Input: part model. Units: mm. Frame: model coordinates. Face numbers are marked on the shaded views. A direction names the side the tool comes from. Round coordinates to 2 decimals unless told otherwise and drop trailing zeros. Loops run counter-clockwise (first coordinate to the right, second up) from the corner with the lowest first, then second, coordinate; pieces in that order, holes last. Notation, with made-up numbers: M 39.25,21 L 49.25,21 A7 ccw 49.25,30 Z; hole C 9.25,-1 d7. An arc over 180 degrees is marked long. Put each result on its own line as item: value. Start each with the question number.
1) Section A-A on x = -5. Output: boundary loops of the cut face in (y, z).
2) Draft query along X for the marked faces 3, 4, 5 and 6. Return one class per face: +X half, -X half, draft (parallel to the pull), parting line (faces both ways), or undercut.
3) Section B-B on z = 32.5. Output: boundary loops of the cut face in (x, y), plus the area to 3 significant figures.
4) Section C-C on y = -8. Output: boundary loops of the cut face in (x, z), plus the area to 3 significant figures.
5) Reachability of the marked faces 1 and 2 from +Z, -Z, +X, -X, +Y, -Y: full face, straight path, thin tool, end or side. Return the list, or none.
6) Line query: probe 1 along Y at (x, z) = (-5, 4); probe 2 along Y at (x, z) = (95.25, 48.2) (3 decimals); probe 3 along X at (y, z) = (-8.5, 38.5). Output: solid intervals per line, ascending.
7) Pin query (flat end, axial travel): pin 1 (5 mm diameter, centred on y = -27, z = 25.7, fed in from -X); pin 2 (6.5 mm diameter, centred on x = -5, y = -15.2, fed in from +Z); pin 3 (4.5 mm diameter, centred on y = 25, z = 48.2, fed in from +X); pin 4 (3 mm diameter, centred on y = 8.5, z = 6.5, fed in from +X). Return the tip coordinate at first contact, or that it passes through.
8) Section D-D on z = 48.2. Output: boundary loops of the cut face in (x, y) (3 decimals).
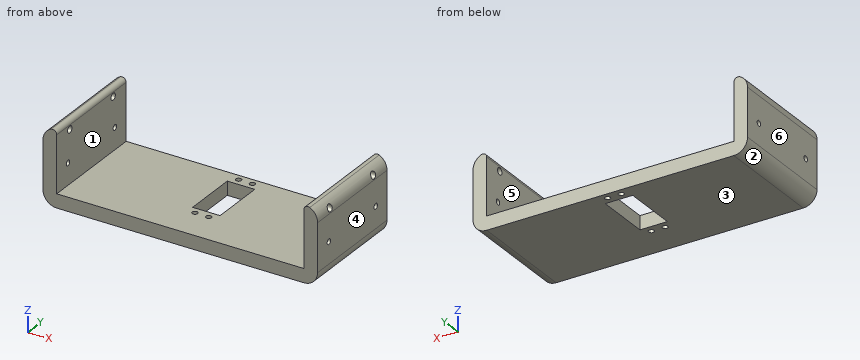
from build123d import *

# Parameters (mm, degrees)
ESQUISSE1_W             = 200
ESQUISSE1_H             = 80
BOSS_EXTRU_1_DEPTH      = 10
ESQUISSE2_W             = 10
ESQUISSE2_H             = 80
BOSS_EXTRU_2_DEPTH      = 50
ESQUISSE8_R             = 2
ENL_V_MAT_EXTRU_3_DEPTH = 213.602916255
ESQUISSE9_W             = 10
ESQUISSE9_H             = 80
ENL_V_MAT_EXTRU_4_DEPTH = 5
ESQUISSE10_R            = 2.515
ENL_V_MAT_EXTRU_5_DEPTH = 202.804360706
ENL_V_START             = -5
ESQUISSE11_R            = 2.515
ENL_V_MAT_EXTRU_6_DEPTH = 5
CONG_1_R                = 10
CONG_2_START            = -41
CONG_2_DEPTH            = 82
CONG_3_R                = 3
ESQUISSE12_W            = 20
ESQUISSE12_H            = 40
ENL_V_MAT_EXTRU_7_DEPTH = 121.628178046
ESQUISSE13_R            = 2
ENL_V_MAT_EXTRU_8_DEPTH = 117.467447093
ESQUISSE14_R            = 2
ENL_V_MAT_EXTRU_9_DEPTH = 212.071450838


with BuildPart() as part:
    # Esquisse1 → Boss.-Extru.1 (new body)
    with BuildSketch(Plane.XY):
        Rectangle(ESQUISSE1_W, ESQUISSE1_H)
    extrude(amount=BOSS_EXTRU_1_DEPTH)

    # Esquisse2 → Boss.-Extru.2 (add)
    with BuildSketch(Plane.XY.offset(10)):
        with Locations((-95, 0)):
            Rectangle(ESQUISSE2_W, ESQUISSE2_H)
        with Locations((95, 0)):
            Rectangle(ESQUISSE2_W, ESQUISSE2_H)
    extrude(amount=BOSS_EXTRU_2_DEPTH)

    # Esquisse8 → Enlèv. mat.-Extru.3 (cut, through all)
    with BuildSketch(Plane(origin=(100, 0, 0), x_dir=(0, 0, -1), z_dir=(1, 0, 0))):
        with Locations(Location((-25.7, 27, 0), (0, 0, 90))):
            Circle(ESQUISSE8_R)
    extrude(amount=-ENL_V_MAT_EXTRU_3_DEPTH, mode=Mode.SUBTRACT)

    # Esquisse9 → Enlèv. mat.-Extru.4 (cut)
    with BuildSketch(Plane.XY.offset(60)):
        with Locations((-95, 0)):
            Rectangle(ESQUISSE9_W, ESQUISSE9_H)
        with Locations((95, 0)):
            Rectangle(ESQUISSE9_W, ESQUISSE9_H)
    extrude(amount=-ENL_V_MAT_EXTRU_4_DEPTH, mode=Mode.SUBTRACT)

    # Esquisse10 → Enlèv. mat.-Extru.5 (cut, through all)
    with BuildSketch(Plane.ZY.offset(-90)):
        with Locations(Location((48.2, 25, 0), (0, 0, 270))):
            Circle(ESQUISSE10_R)
        with Locations(Location((48.2, -25, 0), (0, 0, 270))):
            Circle(ESQUISSE10_R)
    extrude(amount=-ENL_V_MAT_EXTRU_5_DEPTH, mode=Mode.SUBTRACT)

    # Esquisse11 → Enlèv. mat.-Extru.6 (cut)
    with BuildSketch(Plane.ZY.offset(100).offset(ENL_V_START)):
        with Locations(Location((48.2, 25, 0), (0, 0, 270))):
            Circle(ESQUISSE11_R)
        with Locations(Location((48.2, -25, 0), (0, 0, 270))):
            Circle(ESQUISSE11_R)
    extrude(amount=-ENL_V_MAT_EXTRU_6_DEPTH, mode=Mode.SUBTRACT)

    # Congé1
    cong_1_edges = [part.edges().sort_by_distance(p)[0] for p in [
        (-100, 0, 0),
        (100, 0, 0),
    ]]
    fillet(cong_1_edges, radius=CONG_1_R)

    # Congé2: read off the stored shape, not the designer's step
    # Congé2 outline → Congé2 (cut)
    with BuildSketch(Plane(origin=(0, 0, 0), x_dir=(1, 0, 0), z_dir=(0, 1, 0)).offset(CONG_2_START)):
        with BuildLine():
            Line((100, -55), (100, -45))
            ThreePointArc((100, -45), (97.071067812, -52.071067812), (90, -55))
            Line((90, -55), (100, -55))
        make_face()
        with BuildLine():
            ThreePointArc((-90, -55), (-97.071067812, -52.071067812), (-100, -45))
            Line((-100, -45), (-100, -55))
            Line((-100, -55), (-90, -55))
        make_face()
    extrude(amount=CONG_2_DEPTH, mode=Mode.SUBTRACT)

    # Congé3
    cong_3_edges = [part.edges().sort_by_distance(p)[0] for p in [
        (-90, 0, 55),
        (90, 0, 55),
    ]]
    fillet(cong_3_edges, radius=CONG_3_R)

    # Esquisse12 → Enlèv. mat.-Extru.7 (cut, through all)
    with BuildSketch(Plane(origin=(0, 0, 0), x_dir=(-1, 0, 0), z_dir=(0, 0, -1))):
        with Locations((0, 10)):
            Rectangle(ESQUISSE12_W, ESQUISSE12_H)
    extrude(amount=-ENL_V_MAT_EXTRU_7_DEPTH, mode=Mode.SUBTRACT)

    # Esquisse13 → Enlèv. mat.-Extru.8 (cut, through all)
    with BuildSketch(Plane.XY.offset(10)):
        with Locations((-5, 35.2)):
            Circle(ESQUISSE13_R)
        with Locations((5, 35.2)):
            Circle(ESQUISSE13_R)
        with Locations((-5, -15.2)):
            Circle(ESQUISSE13_R)
        with Locations((5, -15.2)):
            Circle(ESQUISSE13_R)
    extrude(amount=-ENL_V_MAT_EXTRU_8_DEPTH, mode=Mode.SUBTRACT)

    # Esquisse14 → Enlèv. mat.-Extru.9 (cut, through all)
    with BuildSketch(Plane.ZY.offset(100)):
        with Locations(Location((25.7, 27, 0), (0, 0, 90))):
            Circle(ESQUISSE14_R)
        with Locations(Location((25.7, -27, 0), (0, 0, 270))):
            Circle(ESQUISSE14_R)
    extrude(amount=-ENL_V_MAT_EXTRU_9_DEPTH, mode=Mode.SUBTRACT)


solid = part.part
Geometry results:
1. outline: M -40,0 L -17.2,0 L -17.2,10 L -40,10 Z; M -13.2,0 L -10,0 L -10,10 L -13.2,10 Z; M 30,0 L 33.2,0 L 33.2,10 L 30,10 Z; M 37.2,0 L 40,0 L 40,10 L 37.2,10 Z
2. face 3: draft
2. face 4: +X half
2. face 5: undercut
2. face 6: -X half
3. outline: M -100,-40 L -90,-40 L -90,40 L -100,40 Z; M 90,-40 L 100,-40 L 100,40 L 90,40 Z
3. area: 1,600 mm²
4. outline: M -100,10 A10 ccw -90,0 L -10,0 L -10,10 L -90,10 L -90,51.32 A3 ccw -94.29,54.04 A10 ccw -100,45 Z; M 10,0 L 90,0 A10 ccw 100,10 L 100,45 A10 ccw 94.29,54.04 A3 ccw 90,51.32 L 90,10 L 10,10 Z
4. area: 2,610 mm²
5. face 1: +Z, +Y, -Y
5. face 2: -Z, -X, +Y, -Y
6. probe 1: y = -40 to -17.2, -13.2 to -10, 30 to 33.2, 37.2 to 40
6. probe 2: y = -40 to -27.515, -22.485 to 22.485, 27.515 to 40
6. probe 3: x = -100 to -90, 90 to 100
7. pin 1: stops at x = -100
7. pin 2: stops at z = 10
7. pin 3: stops at x = -95
7. pin 4: stops at x = 99.8
8. outline: M -99.474,-40 L -90,-40 L -90,-27.515 L -95,-27.515 L -95,-22.485 L -90,-22.485 L -90,22.485 L -95,22.485 L -95,27.515 L -90,27.515 L -90,40 L -99.474,40 Z; M 90,-40 L 99.474,-40 L 99.474,-27.515 L 90,-27.515 Z; M 90,-22.485 L 99.474,-22.485 L 99.474,22.485 L 90,22.485 Z; M 90,27.515 L 99.474,27.515 L 99.474,40 L 90,40 Z
